Read the model definition and answer for the solid it produces. Units are mm, in the model's axes. Give positions to 0.01 mm unless a question says otherwise; leave off trailing zeros. Order: outer loops, then holes, each group sorted by start corner. A loop starts at its lowest first (then second) coordinate and runs counter-clockwise, first axis right, second up. Notation, with made-up numbers: (51, 38.25) - (59, 38.25) arc R23 ccw to (59, 63.25) - close; hole circle Ø7 at (71, 20). An arc over 180 degrees is marked (long way). One line per item, written item: value. Start each with the question number.
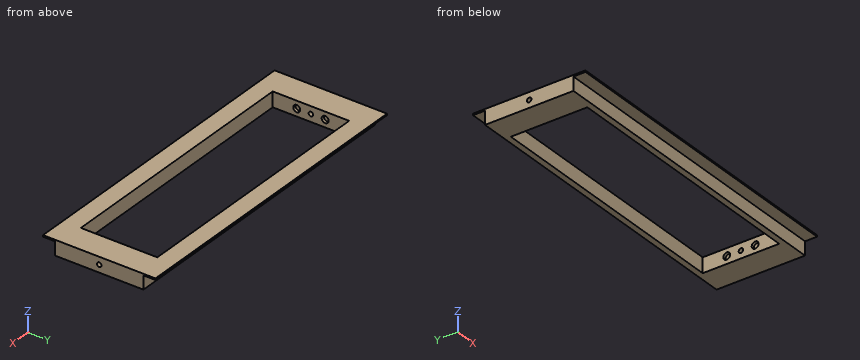
```python
from build123d import *

# Parameters (mm, degrees)
F0_W      = 266.5222
F0_H      = 95.1992
F1_DEPTH  = 12.7
F2_W      = 220.8022
F2_H      = 64.7192
F2_W_2    = 215.7222
F2_H_2    = 44.3992
F3_DEPTH  = 25.4
F4_R      = 1.905
F5_DEPTH  = 508
F6_R      = 2.921
F7_DEPTH  = 2.5146
F8_R      = 2.921
F9_DEPTH  = 2.5146
F10_W     = 10.16
F10_H     = 11.43
F11_DEPTH = 508


with BuildPart() as f1:
    # F0 (on Top) → F1 (new body)
    with BuildSketch(Plane.XY):
        Rectangle(F0_W, F0_H)
    extrude(amount=F1_DEPTH)

    # F2 (on face) → F3 (cut)
    with BuildSketch(Plane.XY.offset(12.7)):
        Rectangle(F2_W, F2_H)
        Rectangle(F2_W_2, F2_H_2, mode=Mode.SUBTRACT)
        Rectangle(F2_W_2, F2_H_2)
    extrude(amount=-F3_DEPTH, mode=Mode.SUBTRACT)

    # F4 (on face) → F5 (cut)
    with BuildSketch(Plane.YZ.offset(133.2611)):
        with Locations((0, 6.35)):
            Circle(F4_R)
    extrude(amount=-F5_DEPTH, mode=Mode.SUBTRACT)

    # F6 (on face) → F7 (cut)
    with BuildSketch(Plane.YZ.offset(-110.4011)):
        with Locations((-12.0396, 6.35)):
            Circle(F6_R)
        with Locations((12.0396, 6.35)):
            Circle(F6_R)
    extrude(amount=-F7_DEPTH, mode=Mode.SUBTRACT)

    # F8 (on face) → F9 (cut)
    with BuildSketch(Plane(origin=(110.4011, 0, 0), x_dir=(0, -1, 0), z_dir=(-1, 0, 0))):
        with Locations((-12.0396, 6.35)):
            Circle(F8_R)
        with Locations((12.0396, 6.35)):
            Circle(F8_R)
    extrude(amount=-F9_DEPTH, mode=Mode.SUBTRACT)

    # F10 (on face) → F11 (cut)
    with BuildSketch(Plane.YZ.offset(133.2611)):
        with Locations((-42.5196, 5.715)):
            Rectangle(F10_W, F10_H)
        with Locations((42.5196, 5.715)):
            Rectangle(F10_W, F10_H)
    extrude(amount=-F11_DEPTH, mode=Mode.SUBTRACT)


solid = f1.part
```
1) Section B-B on y = 23.5 is taken. Write down the section's boundary in (x, z).
2) Section A-A on x = 41 is taken. Write down the section's boundary in (y, z).
3) Each of these flat-tipped pins is pushed along its axis until it touches: pin 1 (4 mm diameter, centred on x = -48.5, z = 3.5, fed in from -Y); pin 2 (4 mm diameter, centred on x = -6.5, z = 8, fed in from +Y); pin 3 (11 mm diameter, centred on x = -22.5, y = 44, fed in from -Z). Where does it stop, or does it pass through?
4) Section C-C on y = 41.5 is taken. Write down the section's boundary in (x, z).
5) Find the intervals of material crossed by probe 1 along Y at (x, z) = (116, 6.5); probe 2 along Z at (x, y) = (-118.5, 0) (3 decimals); probe 3 along Y at (x, z) = (-4.5, 5.75), in increasing order. Write a range as from..to.
Solved:
1. outline: (-133.26, 0) - (-110.4, 0) - (-110.4, 12.7) - (-133.26, 12.7) - close; (110.4, 0) - (133.26, 0) - (133.26, 12.7) - (110.4, 12.7) - close
2. outline: (-47.6, 11.43) - (-37.44, 11.43) - (-37.44, 0) - (-32.36, 0) - (-32.36, 12.7) - (-47.6, 12.7) - close; (32.36, 0) - (37.44, 0) - (37.44, 11.43) - (47.6, 11.43) - (47.6, 12.7) - (32.36, 12.7) - close
3. pin 1: stops at y = -37.44
3. pin 2: stops at y = 37.44
3. pin 3: stops at z = 11.43
4. outline: (-133.26, 11.43) - (133.26, 11.43) - (133.26, 12.7) - (-133.26, 12.7) - close
5. probe 1: y = -37.44..-1.9, 1.9..37.44
5. probe 2: z = 0..4.445, 8.255..12.7
5. probe 3: y = -37.44..-32.36, 32.36..37.44
